Part model, mm, in its own coordinate system. Give positions to 0.01 mm unless a question says otherwise; leave off trailing zeros. Order: outer loops, then holes, each group sorted by start corner. A loop starts at its lowest first (then second) coordinate and runs counter-clockwise, first axis right, second up. Notation, with made-up numbers: M 50,-1.5 L 107,-1.5 A22 ccw 107,12.5 Z; hole C 35,8.5 d6. An arc over 180 degrees is marked long. Answer as a JSON object with one key per item and string values.
Autodesk Inventor part; units mm, degrees
ref_plane "YZ Plane" through (0, 0, 0) normal (1, 0, 0) x (0, 1, 0)
ref_plane "XZ Plane" through (0, 0, 0) normal (0, 1, 0) x (-1, 0, 0)
ref_plane "XY Plane" through (0, 0, 0) normal (0, 0, 1) x (1, 0, 0)
sketch "スケッチ1" plane through (0, 0, 0) normal (1, 0, 0) x (0, 1, 0)
  circle A0 centre (75.1066, 546.1804) radius 20
  line L0 (398.3077, -642.9996) -> (12.4603, 659.0318)
  line L1 (-81.8954, -654.6507) -> (-61.8954, -654.6507)
  line L2 (-6.7154, 653.3493) -> (379.132, -648.6822)
  line L3 (23.4023, 551.7179) -> (69.424, 565.3561)
  line L4 (34.7675, 513.3665) -> (80.7892, 527.0047)
  circle A1 centre (75.1066, 546.1804) radius 11
  line L5 (12.4603, 659.0318) -> (-6.7154, 653.3493)
  circle A2 centre (35.8315, 544.9714) radius 1.5
  circle A3 centre (41.514, 525.7956) radius 1.5
  point P0 (0, 0)
  point P1 (-384.8954, -222.3173)
  dimension "d0" = 40
  dimension "d1" = 28
  dimension "d2" = 22
  dimension "d3" = 106
  dimension "d4" = 3
  dimension "d5" = 3
  dimension "d6" = 10
  dimension "d7" = 10
  dimension "d8" = 10
  dimension "d9" = 20
extrude "押し出し1" add sketch "スケッチ1" against normal blind 2 contours A0 | A0 L4 L0 L3 | L0 L4 L2 L3
fillet "フィレット1" radius 2 2 edges at (-1, 23.4023, 551.7179) (-1, 34.7675, 513.3665)
equation "\"d7\" = d6"
equation "\"d8\" = d6"
properties part number "dribl-v1-Plate-13" material "アルミニウム 6061"
1. Pin check, flat tips, straight feed: P1, Ø8, axis at y = 81, z = 548.5, coming from the -X side; P2, Ø1, axis at x = -1.5, z = 547.5, coming from the -Y side. Stop position of each tip, or through.
Worked answers:
{"P1": "passes through", "P2": "stops at y = 24.5"}
2. Cut at B-B on z = 549. Give the cut face in (x, y).
Worked answers:
{"outline": "M -2,24.21 L 0,24.21 L 0,64.47 L -2,64.47 Z; M -2,85.74 L 0,85.74 L 0,94.91 L -2,94.91 Z"}
3. Two-plate mould, pull along Z, no slides. Class faces 1 (the cylindrical face through (-0.986, 94.403, 551.44)), 2 (the flat face through (-2, 59, 540)), 3 (the cylindrical face through (-0.986, 41.319, 527.283)): +Z half, -Z half, draft (parallel to the pull), parting line (faces both ways), or undercut.
Worked answers:
{"face 1": "parting line", "face 2": "draft", "face 3": "undercut"}
4. Cut at D-D on z = 559. Give the cut face in (x, y), plus the area to 3 significant figures.
Worked answers:
{"outline": "M -2,47.98 L 0,47.98 L 0,90.46 L -2,90.46 Z", "area": "85.0 mm^2"}
5. Probe line 1 along Y through (x, z) = (-0.6, 539.5); line 2 along Y through (x, z) = (-0.6, 541); line 3 along Z through (x, y) = (-0.85, 40.5). List the from-to ranges inside material, lowest first.
Worked answers:
{"line 1": "y = 27.02 to 66.37, 83.85 to 93.96", "line 2": "y = 26.58 to 65.4, 84.81 to 94.42", "line 3": "z = 515.07 to 524.69, 526.9 to 556.78"}
6. Cut at A-A on y = 76.5. Give the cut face in (x, z), plus the area to 3 significant figures.
Worked answers:
{"outline": "M -2,525.73 L 0,525.73 L 0,535.27 L -2,535.27 Z; M -2,557.09 L 0,557.09 L 0,566.13 L -2,566.13 Z", "area": "37.2 mm^2"}
7. Cut at C-C on x = -0.7. Give the cut face in (y, z), plus the area to 3 significant figures.
Worked answers:
{"outline": "M 23.97,549.8 L 34.2,515.28 A2 ccw 36.69,513.93 L 80.79,527 A20 ccw 69.42,565.36 L 25.32,552.29 A2 ccw Z; hole C 35.83,544.97 d3; hole C 41.51,525.8 d3; hole C 75.11,546.18 d22", "area": "2,150 mm^2"}
